from build123d import *

# Parameters (mm, degrees)
SKETCH1_W           = 95.25
SKETCH1_H           = 177.8
BOSS_EXTRUDE1_DEPTH = 6.35
SKETCH2_W           = 12.7
SKETCH2_H           = 12.7
CUT_EXTRUDE1_DEPTH  = 7.35
LPATTERN1_COUNT     = 4
LPATTERN1_PITCH     = 25.4
SKETCH3_W           = 12.7
SKETCH3_H           = 6.35
CUT_EXTRUDE2_DEPTH  = 7.35
SKETCH5_W           = 6.35
SKETCH5_H           = 12.7
CUT_EXTRUDE4_DEPTH  = 7.35
LPATTERN2_COUNT     = 4
LPATTERN2_PITCH     = 25.4
SKETCH6_W           = 95.25
SKETCH6_H           = 38.1
CUT_EXTRUDE5_DEPTH  = 7.35
SKETCH7_W           = 12.7
SKETCH7_H           = 6.35
BOSS_EXTRUDE2_DEPTH = 6.35
LPATTERN3_COUNT     = 2
LPATTERN3_PITCH     = 25.4
LPATTERN3_COL_COUNT = 2
LPATTERN3_COL_PITCH = 25.4
LPATTERN4_COUNT     = 2
LPATTERN4_PITCH     = 76.2
SKETCH8_R           = 12.7
CUT_EXTRUDE6_DEPTH  = 7.35


with BuildPart() as part:
    # Sketch1 → Boss-Extrude1 (new body)
    with BuildSketch(Plane.XY):
        with Locations((47.625, 88.9)):
            Rectangle(SKETCH1_W, SKETCH1_H)
    extrude(amount=BOSS_EXTRUDE1_DEPTH)

    # Sketch2 → Cut-Extrude1 (cut, through all)
    with BuildSketch(Plane.XY.offset(6.35)):
        with Locations((6.35, 6.35)):
            Rectangle(SKETCH2_W, SKETCH2_H)
        with Locations((88.9, 6.35)):
            Rectangle(SKETCH2_W, SKETCH2_H)
    cut_extrude1 = extrude(amount=-CUT_EXTRUDE1_DEPTH, mode=Mode.SUBTRACT)

    # LPattern1: Cut-Extrude1 ×4
    with Locations(*[(0, i * LPATTERN1_PITCH, 0) for i in range(1, LPATTERN1_COUNT)]):
        add(cut_extrude1, mode=Mode.SUBTRACT)

    # Sketch3 → Cut-Extrude2 (cut, through all)
    with BuildSketch(Plane.XY.offset(6.35)):
        with Locations((34.925, 41.275)):
            Rectangle(SKETCH3_W, SKETCH3_H)
        with Locations((60.325, 41.275)):
            Rectangle(SKETCH3_W, SKETCH3_H)
    cut_extrude2 = extrude(amount=-CUT_EXTRUDE2_DEPTH, mode=Mode.SUBTRACT)

    # Sketch5 → Cut-Extrude4 (cut, through all)
    with BuildSketch(Plane.XY.offset(6.35)):
        with Locations((3.175, 107.95)):
            Rectangle(SKETCH5_W, SKETCH5_H)
        with Locations((92.075, 107.95)):
            Rectangle(SKETCH5_W, SKETCH5_H)
    cut_extrude4 = extrude(amount=-CUT_EXTRUDE4_DEPTH, mode=Mode.SUBTRACT)

    # LPattern2: Cut-Extrude4 ×4
    with Locations(*[(0, i * LPATTERN2_PITCH, 0) for i in range(1, LPATTERN2_COUNT)]):
        add(cut_extrude4, mode=Mode.SUBTRACT)

    # Sketch6 → Cut-Extrude5 (cut, through all)
    with BuildSketch(Plane.XY.offset(6.35)):
        with Locations((47.625, 158.75)):
            Rectangle(SKETCH6_W, SKETCH6_H)
    extrude(amount=-CUT_EXTRUDE5_DEPTH, mode=Mode.SUBTRACT)

    # Sketch7 → Boss-Extrude2 (add)
    with BuildSketch(Plane(origin=(0, 139.7, 0), x_dir=(1, 0, 0), z_dir=(0, 1, 0))):
        with Locations((47.625, -3.175)):
            Rectangle(SKETCH7_W, SKETCH7_H)
    boss_extrude2 = extrude(amount=BOSS_EXTRUDE2_DEPTH)

    # LPattern3: Boss-Extrude2 ×2
    with Locations(*[(i * LPATTERN3_PITCH, 0, 0) for i in range(1, LPATTERN3_COUNT)]):
        add(boss_extrude2)

    # LPattern3 col: Boss-Extrude2 ×2
    with Locations(*[(-i * LPATTERN3_COL_PITCH, 0, 0) for i in range(1, LPATTERN3_COL_COUNT)]):
        add(boss_extrude2)

    # LPattern4: Cut-Extrude2 ×2
    with Locations(*[(0, i * LPATTERN4_PITCH, 0) for i in range(1, LPATTERN4_COUNT)]):
        add(cut_extrude2, mode=Mode.SUBTRACT)

    # Sketch8 → Cut-Extrude6 (cut, through all)
    with BuildSketch(Plane.XY.offset(6.35)):
        with Locations((47.625, 88.9)):
            Circle(SKETCH8_R)
    extrude(amount=-CUT_EXTRUDE6_DEPTH, mode=Mode.SUBTRACT)


solid = part.part
Verification items for the finished model (mm, model axes). A direction names the side the tool comes from. Give positions to 0.01 mm unless a question says otherwise; leave off trailing zeros. Order: outer loops, then holes, each group sorted by start corner. A loop starts at its lowest first (then second) coordinate and runs counter-clockwise, first axis right, second up. Notation, with made-up numbers: M 9.5,-19.75 L 41.5,-19.75 A19 ccw 41.5,-4.75 Z; hole C 4,-24.5 d1. An arc over 180 degrees is marked long. Answer as a JSON object with one key per item and string values. Group by question number.
1) Mould release check, pull along Y, two halves, no side actions. Record for faces 1 (the face through (0, 95, 3)), 2 (the face through (11, 139.7, 3)), 3 (the face through (28.575, 117, 3)): released by +Y, released by -Y, zero draft, split by the parting line, or undercut.
2) Cross-section at B-B (y = 97). Enter the section's corners in (x, z), then the cut area to 3 significant figures.
3) Cross-section at A-A (x = 87.5). Enter the section's corners in (y, z).
4) Access from +Z, -Z, +X, -X, +Y, -Y to the whole of each face (thin tool, end or side, straight path). Record for faces 4 (the face through (12.7, 57, 3)), 5 (the face through (79.375, 143, 3)), 6 (the face through (89, 25.4, 3)), 7 (the face through (35, 38.1, 3)).
5) Scan lines: line 1 along Y through (x, z) = (29, 6); line 2 along Y through (x, z) = (5, 5.5); line 3 along Y through (x, z) = (83, 2). Record each from-to range of solid material in increasing order. Write a range as [from, to].
6) Cross-section at C-C (z = 4.75). Give the number of separate pieces and of enclosed holes in the cut face, then the cut area to 3 significant figures.
7) Depth check by flat-ended pin: pin 1 Ø3 at (x, z) = (37, 2.5) entering from -Y; pin 2 Ø1.9 at (x, z) = (9, 4.5) entering from +Y; pin 3 Ø3 at (x, z) = (91.5, 3.5) entering from -Y; pin 4 Ø1.5 at (y, z) = (102.5, 5.5) entering from +X. Enter the tip coordinate at first touch or a pass-through.
Result sheet:
{
 "1": {"face 1": "zero draft", "face 2": "released by +Y", "face 3": "undercut"},
 "2": {"outline": "M 0,0 L 37.84,0 L 37.84,6.35 L 0,6.35 Z; M 57.41,0 L 95.25,0 L 95.25,6.35 L 57.41,6.35 Z", "area": "481 mm2"},
 "3": {"outline": "M 12.7,0 L 25.4,0 L 25.4,6.35 L 12.7,6.35 Z; M 38.1,0 L 50.8,0 L 50.8,6.35 L 38.1,6.35 Z; M 63.5,0 L 76.2,0 L 76.2,6.35 L 63.5,6.35 Z; M 88.9,0 L 139.7,0 L 139.7,6.35 L 88.9,6.35 Z"},
 "4": {"face 4": "+Z, -Z, -X", "face 5": "+Z, -Z, +X, +Y", "face 6": "+Z, -Z, +X", "face 7": "+Z, -Z"},
 "5": {"line 1": "y = [0, 38.1], [44.45, 114.3], [120.65, 139.7]", "line 2": "y = [12.7, 25.4], [38.1, 50.8], [63.5, 76.2], [88.9, 101.6], [114.3, 127]", "line 3": "y = [12.7, 25.4], [38.1, 50.8], [63.5, 76.2], [88.9, 139.7]"},
 "6": {"separate pieces": "1", "enclosed holes": "5", "area": "11,100 mm2"},
 "7": {"pin 1": "stops at y = 0", "pin 2": "stops at y = 139.7", "pin 3": "stops at y = 12.7", "pin 4": "stops at x = 88.9"}
}
